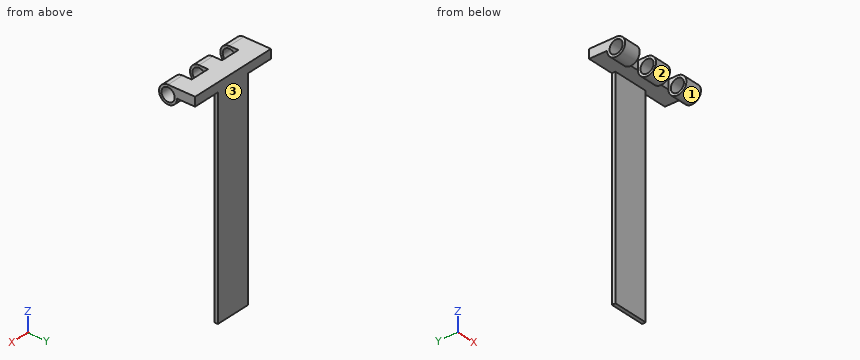
```python
from build123d import *

# Parameters (mm, degrees)
SKETCH1_W               = 6.35
SKETCH1_H               = 19.05
BOSS_EXTRUDE1_DEPTH     = 31.75
SKETCH2_W               = 147.32
SKETCH2_H               = 2.54
EXTRUDE_THIN1_DEPTH     = 12.7
SKETCH3_R               = 6.35
SKETCH4_R               = 4.6355
CUT_EXTRUDE2_DEPTH      = 162.549790777
CUT_EXTRUDE4_DEPTH      = 159.067814244
CUT_EXTRUDE4_DEPTH_BACK = 159.067814244
SKETCH5_W               = 13.716
SKETCH5_H               = 12.7


with BuildPart() as part:
    # Sketch1 → Boss-Extrude1 (new, symmetric)
    with BuildSketch(Plane(origin=(0, 0, 0), x_dir=(0, 0, -1), z_dir=(1, 0, 0))):
        with Locations((-3.175, 9.525)):
            Rectangle(SKETCH1_W, SKETCH1_H)
    extrude(amount=BOSS_EXTRUDE1_DEPTH, both=True)

    # Sketch2 → Extrude-Thin1 (add, symmetric)
    with BuildSketch(Plane(origin=(0, 0, 0), x_dir=(0, 0, -1), z_dir=(1, 0, 0))):
        with Locations((73.66, 17.78)):
            Rectangle(SKETCH2_W, SKETCH2_H)
    extrude(amount=EXTRUDE_THIN1_DEPTH, both=True)

    # Sweep1: sweep along a curve in space
    with BuildLine() as sweep1_path:
        Line((31.75, 0, 0), (-31.75, 0, 0))
    # Sketch3 → Sweep1 (sweep)
    with BuildSketch(Plane(origin=(31.75, 0, 0), x_dir=(0, 0, -1), z_dir=(1, 0, 0))):
        Circle(SKETCH3_R)
    sweep(path=sweep1_path.line)

    # Sketch4 → Cut-Extrude2 (cut, through all)
    with BuildSketch(Plane(origin=(31.75, 0, 0), x_dir=(0, 0, -1), z_dir=(1, 0, 0))):
        Circle(SKETCH4_R)
    extrude(amount=-CUT_EXTRUDE2_DEPTH, mode=Mode.SUBTRACT)

    # Sketch5 → Cut-Extrude4 (cut, two sides: drawn at the far end of the back side and taken through both)
    with BuildSketch(Plane.XY.offset(6.35).offset(-CUT_EXTRUDE4_DEPTH_BACK)):
        with Locations((12.7, 0)):
            Rectangle(SKETCH5_W, SKETCH5_H)
        with Locations((-12.7, 0)):
            Rectangle(SKETCH5_W, SKETCH5_H)
    extrude(amount=CUT_EXTRUDE4_DEPTH + CUT_EXTRUDE4_DEPTH_BACK, mode=Mode.SUBTRACT)


solid = part.part
```
Source: CAD feature listing. Evaluate the final solid. Frame: model axes, mm. Face numbers are marked on the shaded views. Round coordinates to 2 decimals unless told otherwise and drop trailing zeros. Write each loop counter-clockwise with the first axis right and the second up, starting at its lowest first coordinate (ties: lowest second). Pieces come first, ordered by that corner, then holes. Notation, with made-up numbers: M -14,17.5 L 39,17.5 A34 cw 39,56.5 Z; hole C 3,47.25 d8. An arc over 180 degrees is marked long. Use CSV: the item, a comma, the result in double quotes. Start each with the question number.
Q1. Cut plane C-C on x = -3.5. Output: boundary loops of the cut face in (y, z), plus the area to 3 significant figures.
Q2. Cut plane A-A on x = -26. Output: boundary loops of the cut face in (y, z).
Q3. Cut plane B-B on z = -41. Output: boundary loops of the cut face in (x, y).
Q4. Line query: line 1 (X direction, y = -3.5, z = -5); line 2 (Z direction, x = 21.5, y = 13.25); line 3 (Y direction, x = 11, z = -105). Output: solid intervals per line, ascending. Write a range as from..to.
Q5. Pull-direction query (Y, two-part tool) for the marked faces 1, 2 and 3; classes: +Y half, -Y half, draft (parallel to the pull), parting line (faces both ways), or undercut.
Q6. First-contact query: P1, Ø10, axis at y = -3, z = -1, coming from the +X side; P2, Ø1.3, axis at y = 17.5, z = -48, coming from the +X side; P3, Ø2, axis at y = 18, z = -75, coming from the -X side; P4, Ø5, axis at x = 10.5, z = 3, coming from the -Y side. Flat tips, straight axial feed; report the tip coordinate or a pass-through.
Q7. Cut plane D-D on y = 14.5. Output: boundary loops of the cut face in (x, z).
Results found:
1,outline,"M 0,6.35 A6.35 ccw long 6.35,0 L 16.51,0 L 16.51,-147.32 L 19.05,-147.32 L 19.05,6.35 Z; hole C 0,0 d9.27"
1,area,"523 mm^2"
2,outline,"M 0,6.35 A6.35 ccw long 6.35,0 L 19.05,0 L 19.05,6.35 Z; hole C 0,0 d9.27"
3,outline,"M -12.7,16.51 L 12.7,16.51 L 12.7,19.05 L -12.7,19.05 Z"
4,line 1,"-31.75..-19.56, -5.84..5.84, 19.56..31.75"
4,line 2,"0..6.35"
4,line 3,"16.51..19.05"
5,face 1,"parting line"
5,face 2,"undercut"
5,face 3,"+Y half"
6,P1,"x = 31.75"
6,P2,"x = 12.7"
6,P3,"x = -12.7"
6,P4,"y = 6.35"
7,outline,"M -31.75,0 L 31.75,0 L 31.75,6.35 L -31.75,6.35 Z"
